from build123d import *

# Parameters (mm, degrees)
BOSS_EXTRUDE2_DEPTH     = 9.525
CUT_EXTRUDE2_DEPTH      = 20
CUT_EXTRUDE2_DEPTH_BACK = 20
SKETCH5_R               = 98.25
SKETCH5_W               = 192
SKETCH5_H               = 291
FILLET1_R               = 32


with BuildPart() as part:
    # Sketch3 → Boss-Extrude2 (new body)
    with BuildSketch(Plane.XY):
        with BuildLine():
            ThreePointArc((-128.594557171, -271.683003432), (-117.156149866, -292.20930741), (-98.031335876, -305.862431833))
            ThreePointArc((-98.031335876, -305.862431833), (0, -325.672487157), (98.031335876, -305.862431833))
            ThreePointArc((98.031335876, -305.862431833), (117.156149866, -292.20930741), (128.594557171, -271.683003432))
            add(Edge.make_bspline(
                [(128.594557171, -271.683003432), (128.929001137, -270.550670561), (129.607009929, -268.248148567), (132.92675238, -256.894775015), (138.372363082, -237.609630026), (145.587498555, -210.232026724), (152.54164904, -182.662401273), (159.273671104, -155.04724849), (165.68462346, -127.4627227), (173.662799668, -90.634906462), (182.437600317, -44.41870561), (190.23386569, 5.92326819), (194.466912187, 37.721145483), (196.09738159, 50.8)],
                knots=[0.178448909, 0.178448909, 0.178448909, 0.178448909, 0.182331107, 0.186345522, 0.217403108, 0.248460695, 0.279518282, 0.310575869, 0.341633456, 0.372691043, 0.434806217, 0.496921391, 0.540232629, 0.540232629, 0.540232629, 0.540232629], degree=3))
            add(Edge.make_bspline(
                [(196.09738159, 50.8), (196.805263519, 56.478294089), (199.763447664, 80.926441622), (204.336033541, 124.225867737), (208.913068108, 180.752800745), (213.041680781, 256.162202935), (214.132905766, 331.756352431), (212.168857378, 407.250169642), (210.17648868, 444.979630563), (208.923145523, 463.823648231)],
                knots=[0.540232629, 0.540232629, 0.540232629, 0.540232629, 0.559036565, 0.621151739, 0.683266912, 0.745382086, 0.869612434, 0.931727608, 0.993842782, 0.993842782, 0.993842782, 0.993842782], degree=3))
            add(Edge.make_bspline(
                [(208.923145523, 463.823648231), (207.922427582, 478.869564138), (205.602175882, 508.953742276), (199.706639723, 568.910060357), (189.991147, 643.543237919), (177.216824309, 717.777671868), (165.195396161, 776.883168245), (152.011482075, 835.667387937), (133.349255404, 908.643148932), (111.913437805, 980.768947108), (93.147501113, 1037.903472604), (78.26260519, 1080.480419865), (66.491586651, 1112.150932405), (58.40099204, 1133.20563378), (54.364426792, 1143.620772929), (51.51701688, 1150.938010972), (50.030240387, 1154.735608428), (49.858718612, 1155.173455571)],
                knots=[0, 0, 0, 0, 0.062482564, 0.124965127, 0.249930255, 0.374895382, 0.437377946, 0.499860509, 0.624825636, 0.749790764, 0.812273327, 0.874755891, 0.937238455, 0.952859096, 0.968479737, 0.983464396, 0.985416976, 0.985416976, 0.985416976, 0.985416976], degree=3))
            ThreePointArc((49.858718612, 1155.173455571), (0, 1189.189732385), (-49.858718612, 1155.173455571))
            add(Edge.make_bspline(
                [(-208.923145523, 463.823648231), (-207.922427582, 478.869564138), (-205.602175882, 508.953742276), (-199.706639723, 568.910060357), (-189.991147, 643.543237919), (-177.216824309, 717.777671868), (-165.195396161, 776.883168245), (-152.011482075, 835.667387937), (-133.349255404, 908.643148932), (-111.913437805, 980.768947108), (-93.147501113, 1037.903472604), (-78.26260519, 1080.480419865), (-66.491586651, 1112.150932405), (-58.40099204, 1133.20563378), (-54.364426792, 1143.620772929), (-51.51701688, 1150.938010972), (-50.030240387, 1154.735608428), (-49.858718612, 1155.173455571)],
                knots=[0, 0, 0, 0, 0.062482564, 0.124965127, 0.249930255, 0.374895382, 0.437377946, 0.499860509, 0.624825636, 0.749790764, 0.812273327, 0.874755891, 0.937238455, 0.952859096, 0.968479737, 0.983464396, 0.985416976, 0.985416976, 0.985416976, 0.985416976], degree=3))
            add(Edge.make_bspline(
                [(-196.09738159, 50.8), (-196.805263519, 56.478294089), (-199.763447664, 80.926441622), (-204.336033541, 124.225867737), (-208.913068108, 180.752800745), (-213.041680781, 256.162202935), (-214.132905766, 331.756352431), (-212.168857378, 407.250169642), (-210.17648868, 444.979630563), (-208.923145523, 463.823648231)],
                knots=[0.540232629, 0.540232629, 0.540232629, 0.540232629, 0.559036565, 0.621151739, 0.683266912, 0.745382086, 0.869612434, 0.931727608, 0.993842782, 0.993842782, 0.993842782, 0.993842782], degree=3))
            add(Edge.make_bspline(
                [(-128.594557171, -271.683003432), (-128.929001137, -270.550670561), (-129.607009929, -268.248148567), (-132.92675238, -256.894775015), (-138.372363082, -237.609630026), (-145.587498555, -210.232026724), (-152.54164904, -182.662401273), (-159.273671104, -155.04724849), (-165.68462346, -127.4627227), (-173.662799668, -90.634906462), (-182.437600317, -44.41870561), (-190.23386569, 5.92326819), (-194.466912187, 37.721145483), (-196.09738159, 50.8)],
                knots=[0.178448909, 0.178448909, 0.178448909, 0.178448909, 0.182331107, 0.186345522, 0.217403108, 0.248460695, 0.279518282, 0.310575869, 0.341633456, 0.372691043, 0.434806217, 0.496921391, 0.540232629, 0.540232629, 0.540232629, 0.540232629], degree=3))
        make_face()
    extrude(amount=-BOSS_EXTRUDE2_DEPTH)

    # Sketch5 → Cut-Extrude2 (cut, two sides: drawn at the far end of the back side and taken through both)
    with BuildSketch(Plane.XY.offset(-CUT_EXTRUDE2_DEPTH_BACK)):
        with Locations((0, 739.189732385)):
            Circle(SKETCH5_R)
        with Locations((0, -15.172487157)):
            Rectangle(SKETCH5_W, SKETCH5_H)
    extrude(amount=CUT_EXTRUDE2_DEPTH + CUT_EXTRUDE2_DEPTH_BACK, mode=Mode.SUBTRACT)

    # Fillet1
    fillet1_edges = [part.edges().sort_by_distance(p)[0] for p in [
        (-96, -160.672487157, -4.7625),
        (96, -160.672487157, -4.7625),
        (96, 130.327512843, -4.7625),
        (-96, 130.327512843, -4.7625),
    ]]
    fillet(fillet1_edges, radius=FILLET1_R)


solid = part.part
Verification items for the finished model (mm, model axes). A direction names the side the tool comes from. Coordinates: 2 decimals unless noted, no trailing zeros. Write each loop counter-clockwise with the first axis right and the second up, starting at its lowest first coordinate (ties: lowest second). Pieces come first, ordered by that corner, then holes. Notation, with made-up numbers: (38, -30) -> (95, -30) arc R33 ccw to (95, 7) -> close; hole circle Ø4 at (-14, 87). An arc over 180 degrees is marked (long way). One line per item, written item: value. Start each with the question number.
Q1. Access from +Z, -Z, +X, -X, +Y, -Y to the whole of each face (thin tool, end or side, straight path). Record for faces 4 (the cylindrical face through (-117.38, -291.96, -4.7)), 5 (the cylindrical face through (-86.875, 120.705, -4.696)).
Q2. Cross-section at B-B on z = -2.5. State how many separate pieces and enclosed holes the cut face has, and give its area (3 significant figures).
Q3. Cross-section at A-A on x = 0. Enter the section's corners in (y, z) (3 decimals), and give its area (3 significant figures).
Q4. Mould release check, pull along Y, two halves, no side actions. Record for faces 1 (the cylindrical face through (86.377, -151.547, -4.696)), 2 (the cylindrical face through (116.93, -292.46, -4.7)), 3 (the flat face through (-3, 442, -9.525)): pulls with the +Y half, pulls with the -Y half, needs draft (parallel to the pull), parting line crosses it, or undercut.
Q5. Go/stop test with flat-tipped pins: P1, Ø5, axis at y = -45.5, z = -3, coming from the -X side; P2, Ø4, axis at x = 126, z = -5.5, coming from the -Y side; P3, Ø5, axis at x = -33, z = -3.5, coming from the +Y side. Record where each tip stops, or that it passes through.
Q6. Thickness scan on L1, parallel to Y at x = 0, z = -3.5; L2, parallel to Y at x = -33.5, z = -8.5; L3, parallel to X at y = 466, z = -1.75. Record the ranges inside material, lowest first. Write a range as from..to.
Checked values:
1. face 4: +Z, -Z, -X, -Y
1. face 5: +Z, -Z
2. separate pieces: 1
2. enclosed holes: 2
2. area: 413,000 mm²
3. outline: (-325.672, -9.525) -> (-160.672, -9.525) -> (-160.672, 0) -> (-325.672, 0) -> close; (130.328, -9.525) -> (640.94, -9.525) -> (640.94, 0) -> (130.328, 0) -> close; (837.44, -9.525) -> (1189.19, -9.525) -> (1189.19, 0) -> (837.44, 0) -> close
3. area: 9,790 mm²
4. face 1: undercut
4. face 2: pulls with the -Y half
4. face 3: needs draft
5. P1: stops at x = -182.36
5. P2: stops at y = -282.61
5. P3: stops at y = 1179.65
6. L1: y = -325.67..-160.67, 130.33..640.94, 837.44..1189.19
6. L2: y = -323.44..-160.67, 130.33..646.83, 831.55..1177.42
6. L3: x = -208.78..208.78
